Read the model definition and answer for the solid it produces. Units are mm, in the model's axes. Face numbers are marked on the shaded views. A direction names the side the tool comes from. Coordinates: 2 decimals unless noted, no trailing zeros. Loops run counter-clockwise (first coordinate to the right, second up) from the corner with the lowest first, then second, coordinate; pieces in that order, holes last. Notation, with made-up numbers: M 50,53.25 L 92,53.25 A23 cw 92,75.25 Z; hole C 68.5,60 d2. An arc over 180 degrees is marked long. One line per item, written item: value. Start each with the question number.
1. Consider probe 1 along X at (y, z) = (2.55, 0); probe 2 along X at (y, z) = (13.75, 1); probe 3 along Y at (x, z) = (-5, 0). Determine where each line is inside the solid, lowest interval first.
2. The part is cut by section B-B (y = 12). Write down the section's boundary in (x, z), then the cut area to 3 significant figures.
3. Flat-ended cylindrical pins translate along their axes: pin 1 (1.8 mm diameter, centred on y = 12, z = 0, fed in from -X); pin 2 (3 mm diameter, centred on y = 11, z = 0, fed in from +X); pin 3 (3 mm diameter, centred on x = -4, z = -2, fed in from +Y); pin 4 (3 mm diameter, centred on x = -9, z = -0.5, fed in from +Y). Find the tip coordinate at first contact, or state that the pin passes through.
4. The part is cut by section A-A (y = 10). Write down the section's boundary in (x, z).
5. The part is cut by section C-C (x = 7.25). Write down the section's boundary in (y, z), then the cut area to 3 significant figures.
6. For the marked faces 1, 2 and 3, determine the directions among +Z, -Z, +X, -X, +Y, -Y from which every point of the face is accessible in a straight line to the end or side of a thin tool.
7. Determine the mould class of the marked faces 4, 5 and 6 for opening direction X: +X half, -X half, draft (parallel to the pull), parting line (faces both ways), or undercut.
8. The part is cut by section D-D (z = -2.25). Write down the section's boundary in (x, y).
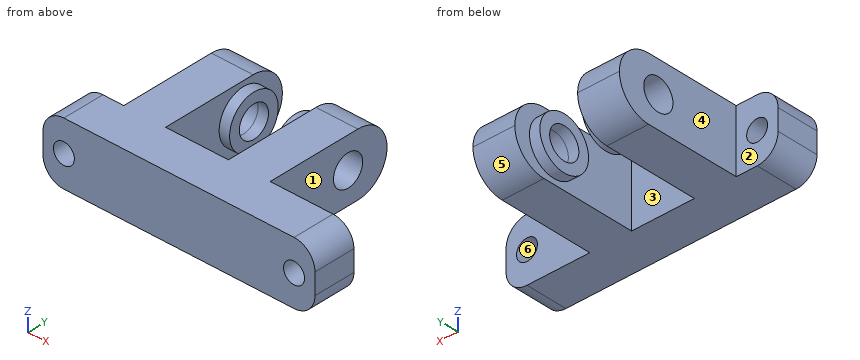
```python
from build123d import *
from build123d.topology import SkipClean

# Parameters (mm, degrees)
SKETCH2_W               = 14
SKETCH2_H               = 6
BOSS_EXTRUDE1_DEPTH     = 4
SKETCH3_W               = 4
SKETCH3_H               = 6
BOSS_EXTRUDE2_DEPTH     = 12
CUT_EXTRUDE1_DEPTH      = 22.470910554
CUT_EXTRUDE1_DEPTH_BACK = 22.470910554
SKETCH4_R               = 1.5
BOSS_EXTRUDE3_START     = 1
SKETCH5_R               = 2.5
SKETCH5_R_2             = 1.5
BOSS_EXTRUDE3_DEPTH     = 1
SKETCH6_R               = 2.5
SKETCH6_R_2             = 1.5
BOSS_EXTRUDE4_DEPTH     = 1
SKETCH7_W               = 8
SKETCH7_H               = 6
SKETCH7_R               = 1
SKETCH7_W_2             = 4
BOSS_EXTRUDE5_DEPTH     = 4
FILLET1_R               = 2
FILLET2_R               = 3


with BuildPart() as part:
    # Sketch2 → Boss-Extrude1 (new body)
    with BuildSketch(Plane(origin=(0, 0, 0), x_dir=(1, 0, 0), z_dir=(0, 1, 0))):
        Rectangle(SKETCH2_W, SKETCH2_H)
    extrude(amount=BOSS_EXTRUDE1_DEPTH)

    # Sketch3 → Boss-Extrude2 (add)
    with BuildSketch(Plane(origin=(0, 4, 0), x_dir=(1, 0, 0), z_dir=(0, 1, 0))):
        with Locations((-5, 0)):
            Rectangle(SKETCH3_W, SKETCH3_H)
        with Locations((5, 0)):
            Rectangle(SKETCH3_W, SKETCH3_H)
    extrude(amount=BOSS_EXTRUDE2_DEPTH)

    # Sketch4 → Cut-Extrude1 (cut, two sides: drawn at the far end of the back side and taken through both)
    with BuildSketch(Plane(origin=(7, 0, 0), x_dir=(0, 0, -1), z_dir=(1, 0, 0)).offset(-CUT_EXTRUDE1_DEPTH_BACK)):
        with Locations((0, 12)):
            Circle(SKETCH4_R)
    extrude(amount=CUT_EXTRUDE1_DEPTH + CUT_EXTRUDE1_DEPTH_BACK, mode=Mode.SUBTRACT)

    # Sketch5 → Boss-Extrude3 (add)
    with BuildSketch(Plane(origin=(-3, 0, 0), x_dir=(0, 0, -1), z_dir=(1, 0, 0)).offset(BOSS_EXTRUDE3_START)):
        with Locations(Location((0, 12, 0), (0, 0, 180))):
            Circle(SKETCH5_R)
        with Locations((0, 12)):
            Circle(SKETCH5_R_2, mode=Mode.SUBTRACT)
    extrude(amount=-BOSS_EXTRUDE3_DEPTH)

    # Sketch6 → Boss-Extrude4 (add)
    with SkipClean():  # the faces are left unmerged after this step: merging them gives an invalid solid
        with BuildSketch(Plane.ZY.offset(-3)):
            with Locations((0, 12)):
                Circle(SKETCH6_R)
            with Locations((0, 12)):
                Circle(SKETCH6_R_2, mode=Mode.SUBTRACT)
        extrude(amount=BOSS_EXTRUDE4_DEPTH)

    # Sketch7 → Boss-Extrude5 (add)
    # profile 1 of 2: a face of its own
    with SkipClean():  # the faces are left unmerged after this step: merging them gives an invalid solid
        with BuildSketch(Plane(origin=(0, 4, 0), x_dir=(1, 0, 0), z_dir=(0, 1, 0))):
            with Locations((11, 0)):
                Rectangle(SKETCH7_W, SKETCH7_H)
            with Locations(Location((13, 0, 0), (0, 0, 270))):
                Circle(SKETCH7_R, mode=Mode.SUBTRACT)
        # profile 2 of 2: a face of its own
        with BuildSketch(Plane(origin=(0, 4, 0), x_dir=(1, 0, 0), z_dir=(0, 1, 0))):
            with Locations((-9, 0)):
                Rectangle(SKETCH7_W_2, SKETCH7_H)
            with Locations(Location((-9, 0, 0), (0, 0, 270))):
                Circle(SKETCH7_R, mode=Mode.SUBTRACT)
        extrude(amount=-BOSS_EXTRUDE5_DEPTH)

    # Fillet1
    fillet1_edges = [part.edges().sort_by_distance(p)[0] for p in [
        (15, 2, -3),
        (15, 2, 3),
        (-11, 2, 3),
        (-11, 2, -3),
    ]]
    fillet(fillet1_edges, radius=FILLET1_R)

    # Fillet2
    fillet2_edges = [part.edges().sort_by_distance(p)[0] for p in [
        (-5, 16, -3),
        (5, 16, -3),
        (5, 16, 3),
        (-5, 16, 3),
    ]]
    fillet(fillet2_edges, radius=FILLET2_R - 0.0001)  # a hair under: the kernel refuses the full size


solid = part.part
```
Answer block:
1. probe 1: x = -11 to -10, -8 to 12, 14 to 15
1. probe 2: x = -7 to -2, 2 to 7
1. probe 3: y = 0 to 10.5, 13.5 to 16
2. outline: M -7,-3 L -3,-3 L -3,-2.5 L -2,-2.5 L -2,-1.5 L -7,-1.5 Z; M -7,1.5 L -2,1.5 L -2,2.5 L -3,2.5 L -3,3 L -7,3 Z; M 2,-2.5 L 3,-2.5 L 3,-3 L 7,-3 L 7,-1.5 L 2,-1.5 Z; M 2,1.5 L 7,1.5 L 7,3 L 3,3 L 3,2.5 L 2,2.5 Z
2. area: 28.0 mm2
3. pin 1: passes through
3. pin 2: stops at x = 7
3. pin 3: stops at y = 15.96
3. pin 4: stops at y = 4
4. outline: M -7,-3 L -3,-3 L -3,-1.5 L -2,-1.5 L -2,1.5 L -3,1.5 L -3,3 L -7,3 Z; M 2,-1.5 L 3,-1.5 L 3,-3 L 7,-3 L 7,3 L 3,3 L 3,1.5 L 2,1.5 Z
5. outline: M 0,-3 L 4,-3 L 4,3 L 0,3 Z
5. area: 24.0 mm2
6. face 1: +Z, -Z, +X, +Y
6. face 2: +Z, -Z, -X, +Y
6. face 3: +Z, -Z
7. face 4: -X half
7. face 5: draft
7. face 6: undercut
8. outline: M -10.56,0 L 14.56,0 L 14.56,4 L 7,4 L 7,14.98 L 3,14.98 L 3,13.09 L 2,13.09 L 2,10.91 L 3,10.91 L 3,4 L -3,4 L -3,10.91 L -2,10.91 L -2,13.09 L -3,13.09 L -3,14.98 L -7,14.98 L -7,4 L -10.56,4 Z
